```python
from build123d import *

# Parameters (mm, degrees)
F0_W     = 0.7586409766
F0_H     = 4.9999998882
F0_H_2   = 9
F0_H_3   = 6.0000001118
F1_ANGLE = 180
F0_W_2   = 1.6913590234
F4_DEPTH = 20
F5_R     = 0.5


with BuildPart() as f1:
    # F0 (on Top) → F1 (revolve)
    with BuildSketch(Plane.XY):
        Polygon((-4, -8.8572846726), (-1.1, -12), (-1.1, 0), (-1.55, 0), (-3.2413590234, 0), (-4, 0), align=None)
        with Locations((-3.6206795117, 2.4999999441)):
            Rectangle(F0_W, F0_H)
        with Locations((-3.6206795117, 9.4999998882)):
            Rectangle(F0_W, F0_H_2)
        with Locations((-3.6206795117, 16.9999999441)):
            Rectangle(F0_W, F0_H_3)
    revolve(axis=Axis((0, 4.4247480631, 0), (0, -1, 0)), revolution_arc=F1_ANGLE)

    # F0 (on Top) → F2 (revolve)
    with BuildSketch(Plane.XY):
        with Locations((-2.3956795117, 2.4999999441)):
            Rectangle(F0_W_2, F0_H)
        with Locations((-2.3956795117, 16.9999999441)):
            Rectangle(F0_W_2, F0_H_3)
    revolve(axis=Axis((0, 4.4247480631, 0), (0, -1, 0)))

    # F3 (on face) → F4 (join)
    with BuildSketch(Plane(origin=(0, 20, 0), x_dir=(-1, 0, 0), z_dir=(0, 1, 0))):
        with BuildLine():
            ThreePointArc((0, -4), (-2.8284271247, -2.8284271247), (-4, 0))
            Line((-4, 0), (-4, -4))
            Line((-4, -4), (0, -4))
        make_face()
        with BuildLine():
            ThreePointArc((4, 0), (2.8284271247, -2.8284271247), (0, -4))
            Line((0, -4), (4, -4))
            Line((4, -4), (4, 0))
        make_face()
    extrude(amount=-F4_DEPTH)

    # F5
    f5_edges = [f1.edges().sort_by_distance(p)[0] for p in [
        (1.1, -6, 0),
        (-1.1, -6, 0),
        (1.55, 5, 0),
        (1.55, 20, 0),
        (3.241359, 9.5, 0),
        (-3.241359, 9.5, 0),
        (4, 20, -2),
        (-4, 20, -2),
        (4, 0, -2),
        (-4, 0, -2),
    ]]
    fillet(f5_edges, radius=F5_R)


solid = f1.part
```
For this review, take the finished solid that the model builds, in its own axes (mm). A direction names the side the tool comes from. Coordinates: 2 decimals unless noted, no trailing zeros. Write each loop counter-clockwise with the first axis right and the second up, starting at its lowest first coordinate (ties: lowest second). Pieces come first, ordered by that corner, then holes. Notation, with made-up numbers: (51.5, 72.5) - (69.5, 72.5) arc R18 cw to (69.5, 106.5) - close; hole circle Ø8 at (-13.5, -34.75). An arc over 180 degrees is marked (long way). Answer in a Markdown table with one row per item. Add a question column.
Q1. For P1, Ø1.9, axis at x = -1.5, z = 1, coming from the -Y side; P2, Ø0.8, axis at x = 0, z = -1, coming from the +Y side; P3, Ø2.5, axis at x = 2.5, z = -3, coming from the -Y side, all flat-tipped, find the tip position at first contact; note any pin that passes through.
Q2. For probe 1 along Y at (x, z) = (-2, 0.25); probe 2 along Z at (x, y) = (0, 1.5); probe 3 along Z at (x, y) = (3.5, 3), list the stretches that pass through material, from the lowest coordinate up.
Q3. We need section C-C, the plane y = -8. State the section outline as (x, z) points, and give its area (3 significant figures).
Q4. We need section D-D, the plane z = 0.75. Count the separate pieces of the cut face and the enclosed holes in it, and give its area (3 significant figures).
Q5. We need section B-B, the plane y = 10. State the section outline as (x, z) points.
Q6. Tool access review of faces 1 (the cylindrical face through (0, -4, -4)), 2 (the cylindrical face through (-0.715, 2.281, 1.375)), 3 (the flat face through (-2, 14, 0)): name each direction out of +Z, -Z, +X, -X, +Y, -Y from which nothing blocks a thin tool from reaching the whole face with its end or side.
Q7. We need section A-A, the plane z = 2.5. State the section outline as (x, y) points.
Q8. Draft analysis for pull direction X (two halves, no side actions). For faces 4 (the conical face through (-0.049, -10.8, -2.207)), 5 (the flat face through (3, 0, -3)), 6 (the cylindrical face through (-0.07, 9.56, -3.24)), state which applies: +X half, -X half, draft (parallel to the pull), parting line (faces both ways), or undercut.
Answer list:
| question | item | result |
|---|---|---|
| 1 | P1 | stops at y = 0 |
| 1 | P2 | stops at y = 0 |
| 1 | P3 | stops at y = -10.31 |
| 2 | probe 1 | y = 0 to 5, 14 to 20 |
| 2 | probe 2 | z = -4 to -1.55, 1.55 to 3.24 |
| 2 | probe 3 | z = -4 to 0 |
| 3 | outline | (-4, 0) arc R4 ccw to (4, 0) - (1.52, 0) arc R0.5 ccw to (1.04, -0.34) arc R1.1 cw to (-1.04, -0.34) arc R0.5 ccw to (-1.52, 0) - close |
| 3 | area | 23.2 mm2 |
| 4 | separate pieces | 4 |
| 4 | enclosed holes | 0 |
| 4 | area | 39.3 mm2 |
| 5 | outline | (-4, -4) - (4, -4) - (4, 0) - (3.71, 0) arc R0.5 ccw to (3.21, -0.43) arc R3.24 cw to (-3.21, -0.43) arc R0.5 ccw to (-3.71, 0) - (-4, 0) - close |
| 6 | face 1 | -Z, -Y |
| 6 | face 2 | +Y |
| 6 | face 3 | +Z |
| 7 | outline | (-2.06, 0) - (2.06, 0) - (2.06, 5) - (-2.06, 5) - close; (-2.06, 14) - (2.06, 14) - (2.06, 20) - (-2.06, 20) - close |
| 8 | face 4 | parting line |
| 8 | face 5 | draft |
| 8 | face 6 | undercut |
